```python
from build123d import *

# Parameters (mm, degrees)
SKETCH_1_W          = 100
SKETCH_1_H          = 100
EXTRUDE_2_DEPTH     = 138.2
SKETCH_1_4_W        = 200
SKETCH_1_4_H        = 200
EXTRUDE_3_DEPTH     = 61.8
SKETCH_1_5_R        = 6.5
CUT_EXTRUDE_1_DEPTH = 177.8


with BuildPart() as part:
    # 草图1 → 凸台-拉伸2 (new body)
    with BuildSketch(Plane.XY):
        with Locations((-2.376531009, -11.802029242)):
            Rectangle(SKETCH_1_W, SKETCH_1_H)
    extrude(amount=EXTRUDE_2_DEPTH)

    # 草图1<4> → 凸台-拉伸3 (add)
    with BuildSketch(Plane.XY):
        with Locations((-2.376531009, -11.802029242)):
            Rectangle(SKETCH_1_4_W, SKETCH_1_4_H)
    extrude(amount=-EXTRUDE_3_DEPTH)

    # 草图1<5> → 切除-拉伸1 (cut)
    with BuildSketch(Plane.XY):
        with Locations((-2.376531009, -11.802029242)):
            Circle(SKETCH_1_5_R)
    extrude(amount=CUT_EXTRUDE_1_DEPTH, mode=Mode.SUBTRACT)


solid = part.part
```
CAD build for the part. Positions are in the model's coordinates, mm. A direction names the side the tool comes from. Round coordinates to 2 decimals unless told otherwise and drop trailing zeros. Order: outer loops, then holes, each group sorted by start corner. A loop starts at its lowest first (then second) coordinate and runs counter-clockwise, first axis right, second up.
Item 1: Probe line 1 along Z through (x, y) = (-75, 20); line 2 along X through (y, z) = (-53, 24); line 3 along X through (y, z) = (-13, 17.5). List the from-to ranges inside material, lowest first.
Item 2: Saw through at A-A on y = 29. Write the cut outline in (x, z), then the cut area to 3 significant figures.
Item 3: Saw through at B-B on x = -46. Write the cut outline in (y, z), then the cut area to 3 significant figures.
Item 4: Pin check, flat tips, straight feed: pin 1 (10 mm diameter, centred on y = -13, z = 22.5, fed in from -X); pin 2 (6 mm diameter, centred on x = 36, y = 55.5, fed in from +Z); pin 3 (12 mm diameter, centred on x = 36.5, z = 70.5, fed in from +Y). Stop position of each tip, or through.
Item 5: Mould opens along Y. For faces 1 (the face through (-4, 88.198, -30)), 2 (the face through (0.62, -17.57, 68.13)), 3 (the face through (-2, -12, 0)), 4 (the face through (47.623, -13, 68)) say: pulls with the +Y half, pulls with the -Y half, needs draft (parallel to the pull), parting line crosses it, or undercut.
Item 6: Saw through at C-C on z = 50.5. Write the cut outline in (x, y).
Item 7: Tool access for faces 5 (the face through (-3, 38.198, 68)), 6 (the face through (-52.377, -13, 68)), 7 (the face through (-3, -61.802, 68)): list every direction of +Z, -Z, +X, -X, +Y, -Y with a clear straight run to the whole face (end or side of a thin tool).
Item 8: Saw through at D-D on y = -76. Write the cut outline in (x, z).
Reported:
1. line 1: z = -61.8 to 0
1. line 2: x = -52.38 to 47.62
1. line 3: x = -52.38 to -8.77, 4.01 to 47.62
2. outline: (-102.38, -61.8) - (97.62, -61.8) - (97.62, 0) - (47.62, 0) - (47.62, 138.2) - (-52.38, 138.2) - (-52.38, 0) - (-102.38, 0) - close
2. area: 26,200 mm2
3. outline: (-111.8, -61.8) - (88.2, -61.8) - (88.2, 0) - (38.2, 0) - (38.2, 138.2) - (-61.8, 138.2) - (-61.8, 0) - (-111.8, 0) - close
3. area: 26,200 mm2
4. pin 1: stops at x = -52.38
4. pin 2: stops at z = 0
4. pin 3: stops at y = 38.2
5. face 1: pulls with the +Y half
5. face 2: undercut
5. face 3: undercut
5. face 4: needs draft
6. outline: (-52.38, -61.8) - (47.62, -61.8) - (47.62, 38.2) - (-52.38, 38.2) - close; hole circle Ø13 at (-2.38, -11.8)
7. face 5: +Z, +X, -X, +Y
7. face 6: +Z, -X, +Y, -Y
7. face 7: +Z, +X, -X, -Y
8. outline: (-102.38, -61.8) - (97.62, -61.8) - (97.62, 0) - (-102.38, 0) - close
